```python
from build123d import *

# Parameters (mm, degrees)
F0_W     = 60
F0_H     = 19
F0_R     = 2.5
F1_DEPTH = 6
F0_H_2   = 5
F2_DEPTH = 20
F4_D     = 5
F5_R     = 5


with BuildPart() as f1:
    # F0 (on Front) → F1 (new body)
    with BuildSketch(Plane.XZ):
        with Locations((0, 2.5)):
            Rectangle(F0_W, F0_H)
        with Locations((-15, -2)):
            Circle(F0_R, mode=Mode.SUBTRACT)
        with Locations((15, -2)):
            Circle(F0_R, mode=Mode.SUBTRACT)
    extrude(amount=F1_DEPTH)

    # F0 (on Front) → F2 (join)
    with BuildSketch(Plane.XZ):
        with Locations((0, -9.5)):
            Rectangle(F0_W, F0_H_2)
    extrude(amount=F2_DEPTH)

    # F4 (through all)
    with Locations(Plane.XY.offset(-7)):
        with Locations((-20, -13), (20, -13)):
            Hole(F4_D / 2)

    # F5
    f5_edges = [f1.edges().sort_by_distance(p)[0] for p in [
        (-30, -3, 12),
        (30, -3, 12),
    ]]
    fillet(f5_edges, radius=F5_R)


solid = f1.part
```
Read the model definition and answer for the solid it produces. Units are mm, in the model's axes. A direction names the side the tool comes from. Coordinates: 2 decimals unless noted, no trailing zeros. Order: outer loops, then holes, each group sorted by start corner. A loop starts at its lowest first (then second) coordinate and runs counter-clockwise, first axis right, second up. Notation, with made-up numbers: (43.5, 43.25) - (82.5, 43.25) arc R19 ccw to (82.5, 61.25) - close; hole circle Ø10 at (-26.5, -20). An arc over 180 degrees is marked (long way). Answer as a JSON object with one key per item and string values. Group by question number.
Item 1: A tool of negligible diameter and unlimited length cuts with its end or side. For faces 1 (the face through (0, -13, -7)), 2 (the face through (0, -20, -9)), from which of +Z, -Z, +X, -X, +Y, -Y can it reach the whole face along a straight path? Write none if from no direction.
Item 2: Section C-C (z = -2) is taken. Give the vertices of the cut face in (x, y), plus the area to 3 significant figures.
Item 3: Flat-ended cylindrical pins translate along their axes: P1, Ø5.5, axis at x = -1, z = 5.5, coming from the -Y side; P2, Ø1.5, axis at x = -16, y = -9, coming from the +Z side; P3, Ø3, axis at x = -15, z = -2, coming from the +Y side. Find the tip coordinate at first contact, or state that the pin passes through.
Item 4: Section A-A (x = 20) is taken. Give the vertices of the cut face in (y, z), plus the area to 3 significant figures.
Item 5: Consider probe 1 along Y at (x, z) = (20, -10.9); probe 2 along Z at (x, y) = (15, -4.2); probe 3 along Z at (x, y) = (15, -10). Determine where each line is inside the solid, lowest interval first. Write a range as from..to.
Item 6: Section B-B (y = -4) is taken. Give the vertices of the cut face in (x, z).
Item 7: Section D-D (z = -8.5) is taken. Give the vertices of the cut face in (x, y), plus the area to 3 significant figures.
Item 8: The mould has two halves that part along X. Classify faces 3 (the face through (0, -6, 3)), 4 (the face through (-29, -3, 10)), 5 (the face through (-18, -14.5, -9.5)), 6 (the face through (30, -5, -5)): +X half, -X half, draft (parallel to the pull), parting line (faces both ways), or undercut.
Results are:
{
 "1": {"face 1": "+Z, +X, -X, -Y", "face 2": "+Z, -Z, +X, -X, -Y"},
 "2": {"outline": "(-30, -6) - (-17.5, -6) - (-17.5, 0) - (-30, 0) - close; (-12.5, -6) - (12.5, -6) - (12.5, 0) - (-12.5, 0) - close; (17.5, -6) - (30, -6) - (30, 0) - (17.5, 0) - close", "area": "300 mm^2"},
 "3": {"P1": "stops at y = -6", "P2": "stops at z = -7", "P3": "passes through"},
 "4": {"outline": "(-20, -12) - (-15.5, -12) - (-15.5, -7) - (-20, -7) - close; (-10.5, -12) - (0, -12) - (0, 12) - (-6, 12) - (-6, -7) - (-10.5, -7) - close", "area": "189 mm^2"},
 "5": {"probe 1": "y = -20..-15.5, -10.5..0", "probe 2": "z = -12..-4.5, 0.5..12", "probe 3": "z = -12..-7"},
 "6": {"outline": "(-30, -12) - (30, -12) - (30, 7) arc R5 ccw to (25, 12) - (-25, 12) arc R5 ccw to (-30, 7) - close; hole circle Ø5 at (-15, -2); hole circle Ø5 at (15, -2)"},
 "7": {"outline": "(-30, -20) - (30, -20) - (30, 0) - (-30, 0) - close; hole circle Ø5 at (-20, -13); hole circle Ø5 at (20, -13)", "area": "1,160 mm^2"},
 "8": {"face 3": "draft", "face 4": "-X half", "face 5": "undercut", "face 6": "+X half"}
}
